Input: part model. Units: mm. Frame: model coordinates. A direction names the side the tool comes from. Coordinates: 2 decimals unless noted, no trailing zeros. Write each loop counter-clockwise with the first axis right and the second up, starting at its lowest first coordinate (ties: lowest second). Pieces come first, ordered by that corner, then holes. Notation, with made-up numbers: (43.25, 63) - (47.25, 63) arc R13 ccw to (47.25, 86) - close; hole circle Ø5 at (7.5, -15.5). An arc over 180 degrees is marked (long way). Put each result on its own line as item: value. Start each with the question number.
1. Cut plane D-D, the plane x = 37.5. Count the separate pieces of the cut face and the enclosed holes in it, and give its area (3 significant figures).
2. Pin query (flat end, axial travel): pin 1 (2.5 mm diameter, centred on x = 88.5, y = 21.5, fed in from -Z); pin 2 (3 mm diameter, centred on x = 27, z = -0.5, fed in from +Y); pin 3 (12 mm diameter, centred on y = 3, z = 5, fed in from -X). Return the tip coordinate at first contact, or that it passes through.
3. Cut plane A-A, the plane x = -9.5. Return loops of the section in (y, z).
4. Access query for faces 4 (the flat face through (59.96, -4, -2)), 5 (the flat face through (90, 20.21, -3)), 6 (the flat face through (36, 26.61, 0)), 7 (the flat face through (84.5, 16, 1)). Directions: +Z, -Z, +X, -X, +Y, -Y. A direction counts if a zero-diameter tool reaches every point of the face in a straight line with its end or side. Return the directions, or none.
5. Line query: line 1 (Z direction, x = 89.5, y = 16); line 2 (X direction, y = 5, z = 3); line 3 (X direction, y = 6, z = -1.25). Output: solid intervals per line, ascending.
6. Cut plane B-B, the plane x = 89.5. Return loops of the section in (y, z).
7. Cut plane C-C, the plane y = -2.5. Return loops of the section in (x, z), and give its area (3 significant figures).
8. Pull-direction query (Z, two-part tool) for faces 1 (the flat face through (4.04, -4, -9)), 2 (the flat face through (-9, -3, -13)), 3 (the cylindrical face through (40.56, 5.73, 0.15)); classes: released by +Z, released by -Z, zero draft, split by the parting line, or undercut.
from build123d import *

# Parameters (mm, degrees)
SKETCH1_R               = 2.16
BOSS_EXTRUDE1_DEPTH     = 26.61
CUT_EXTRUDE1_DEPTH      = 3.5
CUT_EXTRUDE2_DEPTH      = 4
SKETCH5_W               = 110.08
SKETCH5_H               = 13.54
SKETCH5_R               = 2.16
BOSS_EXTRUDE2_DEPTH     = 7
BOSS_EXTRUDE3_DEPTH     = 6.39
BOSS_EXTRUDE4_DEPTH     = 13.54
CUT_EXTRUDE3_START      = -1.4
SKETCH8_R               = 2.16
CUT_EXTRUDE3_DEPTH      = 3.4
CUT_EXTRUDE4_START      = -29.61
SKETCH8_2_R             = 2.16
CUT_EXTRUDE4_DEPTH      = 42
CHAMFER2_SIZE           = 2
SKETCH10_R              = 2.16
CUT_EXTRUDE5_DEPTH      = 1
CUT_EXTRUDE5_DEPTH_BACK = 14.54
SKETCH10_3_R            = 5.196152423
CUT_EXTRUDE6_DEPTH      = 3
SKETCH11_W              = 27.08
SKETCH11_H              = 7
CUT_EXTRUDE7_DEPTH      = 7.5
SKETCH11_3_W            = 27.08
SKETCH11_3_H            = 7
BOSS_EXTRUDE5_DEPTH     = 7.5
SKETCH12_R              = 3.55
CUT_EXTRUDE8_DEPTH      = 7.5


with BuildPart() as part:
    # Sketch1 → Boss-Extrude1 (new body)
    with BuildSketch(Plane(origin=(0, 0, 0), x_dir=(1, 0, 0), z_dir=(0, 1, 0))):
        Polygon((-23.04, -8.04), (-23.04, 5.5), (-20.5, 5.5), (-20.5, -5.5), (20.5, -5.5), (20.5, 5.5), (23.04, 5.5), (40.96, 5.5), (43.5, 5.5), (43.5, -5.5), (84.5, -5.5), (84.5, 5.5), (87.04, 5.5), (87.04, -8.04), (40.96, -8.04), (23.04, -8.04), align=None)
        with Locations((25.5, 0.5)):
            Circle(SKETCH1_R, mode=Mode.SUBTRACT)
        with Locations((38.5, 0.5)):
            Circle(SKETCH1_R, mode=Mode.SUBTRACT)
    extrude(amount=BOSS_EXTRUDE1_DEPTH)

    # Sketch3 → Cut-Extrude1 (cut)
    with BuildSketch(Plane(origin=(0, 21.61, 0), x_dir=(1, 0, 0), z_dir=(0, 1, 0))):
        Polygon((28.098076211, -4), (30.696152423, 0.5), (28.098076211, 5), (27.809401077, 5.5), (20.5, 5.5), (20.5, -4), (22.901923789, -4), align=None)
        Polygon((35.901923789, 5), (33.303847577, 0.5), (35.901923789, -4), (41.098076211, -4), (43.5, -4), (43.5, 5.5), (36.190598923, 5.5), align=None)
    extrude(amount=-CUT_EXTRUDE1_DEPTH, mode=Mode.SUBTRACT)

    # Sketch4 → Cut-Extrude2 (cut)
    with BuildSketch(Plane.ZY.offset(23.04)):
        Polygon((-5.5, 7.5), (2, 0), (-5.5, 0), align=None)
    cut_extrude2 = extrude(amount=-CUT_EXTRUDE2_DEPTH, mode=Mode.SUBTRACT)

    # Mirror1: Cut-Extrude2 across plane
    add(cut_extrude2.mirror(Plane(origin=(32, 0, 0), x_dir=(0, 0, 1), z_dir=(1, 0, 0))), mode=Mode.SUBTRACT)

    # Sketch5 → Boss-Extrude2 (add)
    with BuildSketch(Plane.XZ):
        with Locations((32, 1.27)):
            Rectangle(SKETCH5_W, SKETCH5_H)
        with Locations((38.5, -0.5)):
            Circle(SKETCH5_R, mode=Mode.SUBTRACT)
        with Locations((25.5, -0.5)):
            Circle(SKETCH5_R, mode=Mode.SUBTRACT)
    extrude(amount=BOSS_EXTRUDE2_DEPTH)

    # Sketch6 → Boss-Extrude3 (add)
    with BuildSketch(Plane(origin=(0, 26.61, 0), x_dir=(1, 0, 0), z_dir=(0, 1, 0))):
        Polygon((-23.04, -5.5), (30.5, -5.5), (30.5, 5.5), (33.5, 5.5), (33.5, -5.5), (87.04, -5.5), (87.04, -8.04), (-23.04, -8.04), align=None)
    extrude(amount=BOSS_EXTRUDE3_DEPTH)

    # Sketch7 → Boss-Extrude4 (add)
    with BuildSketch(Plane.XY.offset(8.04)):
        Polygon((-23.04, 26.61), (-31.54, 26.61), (-31.54, 20.11), (-23.04, 11.61), align=None)
    boss_extrude4 = extrude(amount=-BOSS_EXTRUDE4_DEPTH)

    # Sketch8 → Cut-Extrude3 (cut)
    with BuildSketch(Plane(origin=(0, 21.61, 0), x_dir=(1, 0, 0), z_dir=(0, 1, 0)).offset(CUT_EXTRUDE3_START)):
        Polygon((-30.696152423, 0.5), (-31.54, 1.961586878), (-31.54, 5.5), (-20.5, 5.5), (-20.5, 0.160254038), (-22.901923789, -4), (-28.098076211, -4), align=None)
        with Locations((-25.5, 0.5)):
            Circle(SKETCH8_R, mode=Mode.SUBTRACT)
    cut_extrude3 = extrude(amount=CUT_EXTRUDE3_DEPTH, mode=Mode.SUBTRACT)

    # Sketch8<2> → Cut-Extrude4 (cut)
    with BuildSketch(Plane(origin=(0, 21.61, 0), x_dir=(1, 0, 0), z_dir=(0, 1, 0)).offset(CUT_EXTRUDE4_START)):
        with Locations((-25.5, 0.5)):
            Circle(SKETCH8_2_R)
    cut_extrude4 = extrude(amount=CUT_EXTRUDE4_DEPTH, mode=Mode.SUBTRACT)

    # Mirror2: Boss-Extrude4, Cut-Extrude3, Cut-Extrude4 across plane
    add(boss_extrude4.mirror(Plane(origin=(32, 0, 0), x_dir=(0, 0, 1), z_dir=(1, 0, 0))))
    add(cut_extrude3.mirror(Plane(origin=(32, 0, 0), x_dir=(0, 0, 1), z_dir=(1, 0, 0))), mode=Mode.SUBTRACT)
    add(cut_extrude4.mirror(Plane(origin=(32, 0, 0), x_dir=(0, 0, 1), z_dir=(1, 0, 0))), mode=Mode.SUBTRACT)

    # Chamfer2
    chamfer2_edges = [part.edges().sort_by_distance(p)[0] for p in [
        (84.5, 3.75, -1.75),
        (-20.5, 3.75, -1.75),
    ]]
    chamfer(chamfer2_edges, length=CHAMFER2_SIZE)

    # Sketch10 → Cut-Extrude5 (cut, two sides)
    with BuildSketch(Plane.XY.offset(8.04)) as cut_extrude5_sk:
        with Locations((26.5, 9.055)):
            Circle(SKETCH10_R)
        with Locations((37.5, 9.055)):
            Circle(SKETCH10_R)
    extrude(amount=CUT_EXTRUDE5_DEPTH, mode=Mode.SUBTRACT)
    extrude(cut_extrude5_sk.sketch, amount=-CUT_EXTRUDE5_DEPTH_BACK, mode=Mode.SUBTRACT)

    # Sketch10<3> → Cut-Extrude6 (cut)
    with BuildSketch(Plane.XY.offset(8.04)):
        with Locations((26.5, 9.055)):
            Circle(SKETCH10_3_R)
        with Locations((37.5, 9.055)):
            Circle(SKETCH10_3_R)
    extrude(amount=-CUT_EXTRUDE6_DEPTH, mode=Mode.SUBTRACT)

    # Sketch11 → Cut-Extrude7 (cut)
    with BuildSketch(Plane(origin=(0, 0, -5.5), x_dir=(-1, 0, 0), z_dir=(0, 0, -1))):
        with Locations((-73.5, -3.5)):
            Rectangle(SKETCH11_W, SKETCH11_H)
    extrude(amount=-CUT_EXTRUDE7_DEPTH, mode=Mode.SUBTRACT)

    # Sketch11<3> → Boss-Extrude5 (add)
    with BuildSketch(Plane(origin=(0, 0, -5.5), x_dir=(-1, 0, 0), z_dir=(0, 0, -1))):
        with Locations((9.5, -3.5)):
            Rectangle(SKETCH11_3_W, SKETCH11_3_H)
    extrude(amount=BOSS_EXTRUDE5_DEPTH)

    # Sketch12 → Cut-Extrude8 (cut)
    with BuildSketch(Plane.XZ.offset(7)):
        with Locations((-9.5, -5.5)):
            Circle(SKETCH12_R)
    extrude(amount=-CUT_EXTRUDE8_DEPTH, mode=Mode.SUBTRACT)


solid = part.part
Report:
1. separate pieces: 5
1. enclosed holes: 0
1. area: 263 mm^2
2. pin 1: stops at z = 4
2. pin 2: stops at y = 26.61
2. pin 3: stops at x = -23.04
3. outline: (-7, -13) - (0, -13) - (0, -9.05) - (-7, -9.05) - close; (-7, -1.95) - (0, -1.95) - (0, 5.5) - (33, 5.5) - (33, 8.04) - (-7, 8.04) - close
4. face 4: -Z, +X, +Y, -Y
4. face 5: -Z
4. face 6: -Z, +X, +Y
4. face 7: -Z, +Y
5. line 1: z = -5.5 to -2.66, 1.66 to 8.04
5. line 2: x = -23.04 to -20.5, 20.5 to 43.5, 84.5 to 87.04
5. line 3: x = -23.04 to -20.56, 20.5 to 23.47, 27.53 to 36.47, 40.53 to 43.5, 84.56 to 87.04
6. outline: (14.07, -5.5) - (20.21, -5.5) - (20.21, -2.66) - (14.07, -2.66) - close; (14.07, 1.66) - (20.21, 1.66) - (20.21, 4) - (23.61, 4) - (23.61, 1.66) - (26.61, 1.66) - (26.61, 8.04) - (14.07, 8.04) - close; (23.61, -5.5) - (26.61, -5.5) - (26.61, -2.66) - (23.61, -2.66) - close
7. outline: (-23.04, -13) - (4.04, -13) - (4.04, -5.5) - (59.96, -5.5) - (59.96, 2) - (87.04, 2) - (87.04, 8.04) - (-23.04, 8.04) - close; hole circle Ø7.1 at (-9.5, -5.5); hole circle Ø4.32 at (25.5, -0.5); hole circle Ø4.32 at (38.5, -0.5)
7. area: 1,420 mm^2
8. face 1: zero draft
8. face 2: released by -Z
8. face 3: undercut
